Check sheet for the modelled part. Datum: model origin and axes. Units: mm. Round coordinates to 2 decimals unless told otherwise and drop trailing zeros. Loops run counter-clockwise (first coordinate to the right, second up) from the corner with the lowest first, then second, coordinate; pieces in that order, holes last. Notation, with made-up numbers: (75.25, 45) - (111.25, 45) arc R26 ccw to (111.25, 65) - close; hole circle Ø10 at (-9, -4). An arc over 180 degrees is marked (long way). Return JSON: item names as keys, results as strings.
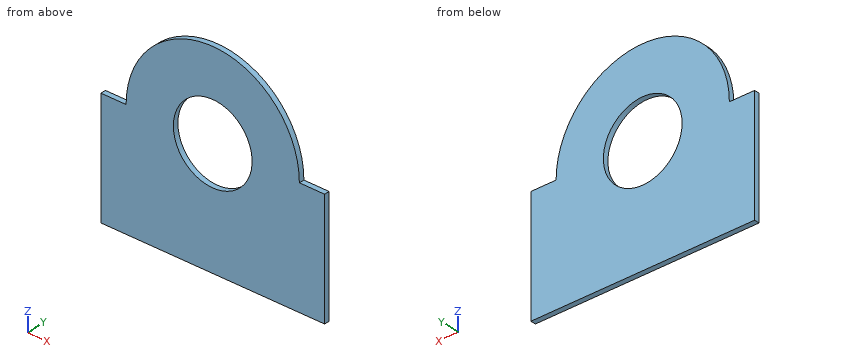
Autodesk Inventor part; units mm, degrees
ref_plane "YZ Plane" through (0, 0, 0) normal (1, 0, 0) x (0, 1, 0)
ref_plane "XZ Plane" through (0, 0, 0) normal (0, 1, 0) x (-1, 0, 0)
ref_plane "XY Plane" through (0, 0, 0) normal (0, 0, 1) x (1, 0, 0)
sketch "Sketch1" plane through (0, 0, 0) normal (0, 1, 0) x (-1, 0, 0)
  line L0 (341.2381, 167.58) -> (341.2381, -52.42)
  line L1 (341.2381, -52.42) -> (-84.7619, -52.42)
  line L2 (-84.7619, -52.42) -> (-84.7619, 167.58)
  arc A0 (293.2381, 167.58) -> (-36.7619, 167.58) centre (128.2381, 167.58) ccw
  line L3 (-84.7619, 167.58) -> (-36.7619, 167.58)
  line L4 (293.2381, 167.58) -> (341.2381, 167.58)
  circle A1 centre (128.2381, 167.58) radius 75
  point P0 (0, 0)
  dimension "d0" = 426
  dimension "d1" = 220
  dimension "d2" = 330
  dimension "d3" = 150
extrude "Extrusion1" add sketch "Sketch1" along normal blind 10
properties part number "frontPlate_half"
Q1. Sectioned sample at C-C (x = -8.5). Enter the section's corners in (y, z), plus the area to 3 significant figures.
Answer key:
{"outline": "(0, -52.42) - (10, -52.42) - (10, 281.1) - (0, 281.1) - close", "area": "3,340 mm²"}
Q2. Depth check by flat-ended pin: P1, Ø4, axis at y = 1.5, z = 208, coming from the +X side. Enter the tip coordinate at first touch or a pass-through.
Answer key:
{"P1": "stops at x = 32.23"}
Q3. Sectioned sample at D-D (z = 305). Enter the section's corners in (x, y), plus the area to 3 significant figures.
Answer key:
{"outline": "(-219.57, 0) - (-36.91, 0) - (-36.91, 10) - (-219.57, 10) - close", "area": "1,830 mm²"}
Q4. Scan lines: probe 1 along X at (y, z) = (5.75, 166); probe 2 along Z at (x, y) = (-307, 6); probe 3 along Z at (x, y) = (-183, 1.5). Record each from-to range of solid material in increasing order. Write a range as [from, to].
Answer key:
{"probe 1": "x = [-341.24, -203.22], [-53.25, 84.76]", "probe 2": "z = [-52.42, 167.58]", "probe 3": "z = [-52.42, 116.33], [218.83, 323.23]"}
Q5. Sectioned sample at A-A (y = 2.5). Enter the section's corners in (x, z).
Answer key:
{"outline": "(-341.24, -52.42) - (84.76, -52.42) - (84.76, 167.58) - (36.76, 167.58) arc R165 ccw to (-293.24, 167.58) - (-341.24, 167.58) - close; hole circle Ø150 at (-128.24, 167.58)"}
Q6. Sectioned sample at B-B (z = 185). Enter the section's corners in (x, y), plus the area to 3 significant figures.
Answer key:
{"outline": "(-292.32, 0) - (-201.19, 0) - (-201.19, 10) - (-292.32, 10) - close; (-55.29, 0) - (35.84, 0) - (35.84, 10) - (-55.29, 10) - close", "area": "1,820 mm²"}
